```python
from build123d import *

# Parameters (mm, degrees)
BOSS_EXTRUDE1_DEPTH = 15
SKETCH6_R           = 26.898177411
CUT_EXTRUDE2_DEPTH  = 9
SKETCH7_W           = 12
SKETCH7_H           = 12
CUT_EXTRUDE3_DEPTH  = 10


with BuildPart() as part:
    # Sketch1 → Boss-Extrude1 (new, symmetric)
    with BuildSketch(Plane(origin=(0, 0, 0), x_dir=(0, 0, -1), z_dir=(1, 0, 0))):
        Polygon((-28, -7), (15, -7), (15, -15.402490459), (-40, -15.402490459), align=None)
    extrude(amount=BOSS_EXTRUDE1_DEPTH, both=True)

    # Sketch6 → Cut-Extrude2 (cut)
    with BuildSketch(Plane(origin=(2.825070642, 7.997590477, 5.599973139), x_dir=(-0.9605940806562516, 0.22768745094625853, 0.1594284695083218), z_dir=(-0.27795505429506184, -0.7868726049014764, -0.5509741295627175))):
        with Locations((-5.77915715, -31.909329579)):
            Circle(SKETCH6_R)
    extrude(amount=-CUT_EXTRUDE2_DEPTH, mode=Mode.SUBTRACT)

    # Sketch7 → Cut-Extrude3 (cut)
    with BuildSketch(Plane.XZ.offset(15.402490459)):
        with Locations((9, -9)):
            Rectangle(SKETCH7_W, SKETCH7_H)
    extrude(amount=-CUT_EXTRUDE3_DEPTH, mode=Mode.SUBTRACT)


solid = part.part
```
Here's how the part is built. I have some questions about the finished solid (model axes, mm). A direction names the side the tool comes from. Coordinates: 2 decimals unless noted, no trailing zeros. Loops run counter-clockwise (first coordinate to the right, second up) from the corner with the lowest first, then second, coordinate; pieces in that order, holes last. Notation, with made-up numbers: (-36, 38) -> (7, 38) arc R24 cw to (7, 69) -> close; hole circle Ø11 at (24.25, 18.25). An arc over 180 degrees is marked (long way). Return JSON: item names as keys, results as strings.
1) If we section it at B-B, the plane z = -9.5: Write out the boundary of the cut face in (x, y), then the cut area to 3 significant figures.
Results below:
{"outline": "(-15, -15.4) -> (3, -15.4) -> (3, -7) -> (-15, -7) -> close", "area": "151 mm²"}
2) If we section it at C-C, the plane x = 8.25: Write out the boundary of the cut face in (y, z), then the cut area to 3 significant figures.
Results below:
{"outline": "(-15.4, -3) -> (-7, -3) -> (-7, 24.28) -> (-15.4, 36.28) -> close", "area": "280 mm²"}
3) If we section it at A-A, the plane y = -10.5: Write out the boundary of the cut face in (x, z), then the cut area to 3 significant figures.
Results below:
{"outline": "(-15, -15) -> (3, -15) -> (3, -3) -> (15, -3) -> (15, 25.88) -> (0.88, 33) -> (-15, 33) -> close", "area": "1,250 mm²"}
4) Will these pins go through, and if not, where does the flat tip stop? pin 1 (3 mm diameter, centred on x = 8, y = -13.5, fed in from +Z); pin 2 (2.5 mm diameter, centred on x = 8, y = -11.5, fed in from -Z).
Results below:
{"pin 1": "z = 35.96", "pin 2": "z = -3"}
5) I need wall thicknesses on line 1 (X direction, y = -9.5, z = -7.5); line 2 (Z direction, x = -6.25, y = -10.25); line 3 (Z direction, x = -8.75, y = -8.5). Which ranges of each line are inside material? Lowest first, please. Write a range as from..to.
Results below:
{"line 1": "-15..3", "line 2": "-15..32.64", "line 3": "-15..30.14"}
6) For faces 1 (the face through (9, -11, -3)), 2 (the face through (8.04, -11.14, 30.3)), which set-ups out of +Z, -Z, +X, -X, +Y, -Y let a thin tool reach every point of the face, with its end or its side?
Results below:
{"face 1": "-Z, +X, +Y, -Y", "face 2": "+Z, +X, +Y"}
7) If we section it at D-D, the plane y = -13.5: Write out the boundary of the cut face in (x, z), then the cut area to 3 significant figures.
Results below:
{"outline": "(-15, -15) -> (3, -15) -> (3, -3) -> (15, -3) -> (15, 30.16) -> (0.88, 37.28) -> (-15, 37.28) -> close", "area": "1,370 mm²"}
